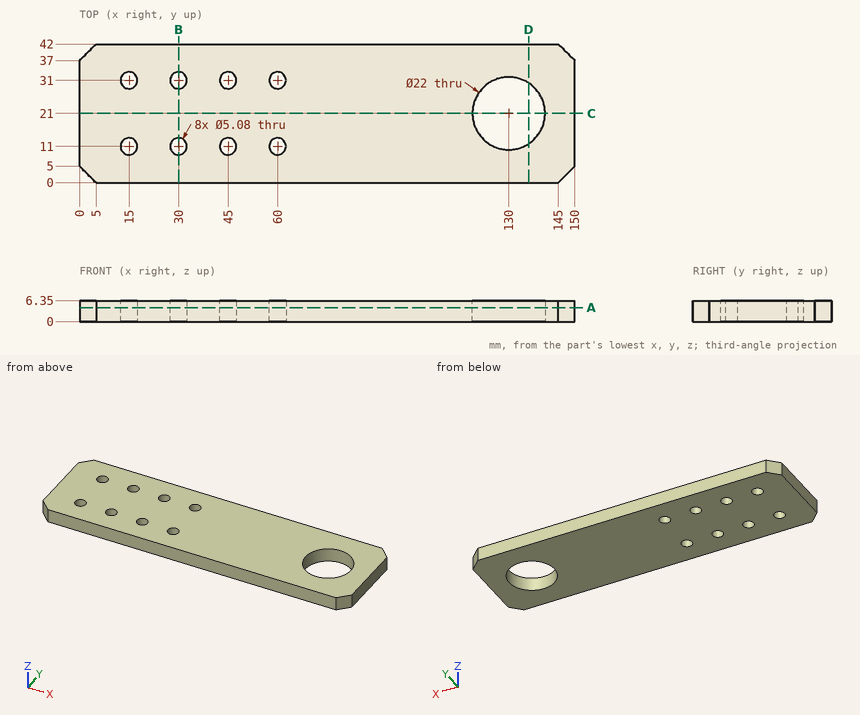
Geometry check sheet. Reference: drawing and pictorial views, mm from the part's lowest x, y, z. Round coordinates to 2 decimals unless told otherwise and drop trailing zeros. Loops run counter-clockwise (first coordinate to the right, second up) from the corner with the lowest first, then second, coordinate; pieces in that order, holes last. Notation, with made-up numbers: (68.25, 40.25) - (88.25, 40.25) arc R22 cw to (88.25, 77.25) - close; hole circle Ø3 at (-14.5, 13). An arc over 180 degrees is marked (long way). Use a Markdown table: item, result. Add a question column.
1. Section check A-A, the plane z = 4.25. Give the number of separate pieces and of enclosed holes in the cut face, plus the area to 3 significant figures.
2. Section check D-D, the plane x = 136. Record the boundary of the cut face in (y, z).
3. Section check C-C, the plane y = 21. Record the boundary of the cut face in (x, z), plus the area to 3 significant figures.
4. Thickness scan on probe 1 along Y at (x, z) = (30, 2); probe 2 along Y at (x, z) = (130, 4.5); probe 3 along X at (y, z) = (20.5, 5). Record the ranges inside material, lowest first. Write a range as [from, to].
5. Section check B-B, the plane x = 30. Record the boundary of the cut face in (y, z).
Checks:
| question | item | result |
|---|---|---|
| 1 | separate pieces | 1 |
| 1 | enclosed holes | 9 |
| 1 | area | 5,710 mm^2 |
| 2 | outline | (0, 0) - (11.78, 0) - (11.78, 6.35) - (0, 6.35) - close; (30.22, 0) - (42, 0) - (42, 6.35) - (30.22, 6.35) - close |
| 3 | outline | (0, 0) - (119, 0) - (119, 6.35) - (0, 6.35) - close; (141, 0) - (150, 0) - (150, 6.35) - (141, 6.35) - close |
| 3 | area | 813 mm^2 |
| 4 | probe 1 | y = [0, 8.46], [13.54, 28.46], [33.54, 42] |
| 4 | probe 2 | y = [0, 10], [32, 42] |
| 4 | probe 3 | x = [0, 119.01], [140.99, 150] |
| 5 | outline | (0, 0) - (8.46, 0) - (8.46, 6.35) - (0, 6.35) - close; (13.54, 0) - (28.46, 0) - (28.46, 6.35) - (13.54, 6.35) - close; (33.54, 0) - (42, 0) - (42, 6.35) - (33.54, 6.35) - close |
